For this review, take the finished solid that the model builds, in its own axes (mm). Face numbers are marked on the shaded views. A direction names the side the tool comes from. Coordinates: 2 decimals unless noted, no trailing zeros. Loops run counter-clockwise (first coordinate to the right, second up) from the corner with the lowest first, then second, coordinate; pieces in that order, holes last. Notation, with made-up numbers: (59, 26.5) -> (88, 26.5) arc R28 cw to (88, 64.5) -> close; hole circle Ø9 at (87.25, 18). An arc over 180 degrees is marked (long way). Use a Markdown table: item, result.
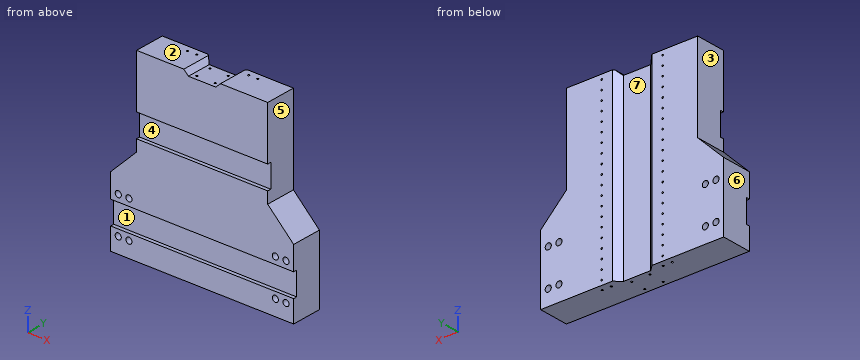
from build123d import *

# Parameters (mm, degrees)
SKETCH1_W                           = 600
SKETCH1_H                           = 600
BOSS_EXTRUDE1_DEPTH                 = 100
CUT_EXTRUDE1_DEPTH                  = 436.889894354
CHAMFER5_SIZE                       = 85
CUT_EXTRUDE2_DEPTH                  = 679.232998313
SKETCH9_R                           = 10
CUT_EXTRUDE5_DEPTH                  = 436.889894354
SKETCH12_R                          = 2.5
CUT_EXTRUDE7_DEPTH                  = 30
SKETCH14_W                          = 90
SKETCH14_H                          = 15
CUT_EXTRUDE8_DEPTH                  = 432.927077179
CHAMFER3_SIZE                       = 15
SKETCH15_W                          = 76.2
SKETCH15_H                          = 12.7
CUT_EXTRUDE9_DEPTH                  = 679.232998313
F_6_0MM_DOWEL_HOLE1_D               = 6
F_6_0MM_DOWEL_HOLE1_DEPTH           = 30
F_6_0MM_DOWEL_HOLE1_TIP             = 1.802581857
F_6_0MM_DOWEL_HOLE1_ON_FACE_2_D     = 6
F_6_0MM_DOWEL_HOLE1_ON_FACE_2_DEPTH = 30
F_6_0MM_DOWEL_HOLE1_ON_FACE_2_TIP   = 1.802581857
F_6_0MM_DOWEL_HOLE1_ON_FACE_3_D     = 6
F_6_0MM_DOWEL_HOLE1_ON_FACE_3_DEPTH = 30
F_6_0MM_DOWEL_HOLE1_ON_FACE_3_TIP   = 1.802581857


with BuildPart() as part:
    # Sketch1 → Boss-Extrude1 (new body)
    with BuildSketch(Plane(origin=(0, 0, 0), x_dir=(1, 0, 0), z_dir=(0, 1, 0))):
        Rectangle(SKETCH1_W, SKETCH1_H)
    extrude(amount=BOSS_EXTRUDE1_DEPTH)

    # Sketch2 → Cut-Extrude1 (cut, through all)
    with BuildSketch(Plane(origin=(0, 100, 0), x_dir=(1, 0, 0), z_dir=(0, 1, 0))):
        Polygon((-300, -300), (-220, -300), (-215, -300), (-215, 74), (-220, 74), (-300, 74), (-300, 60), align=None)
        Polygon((300, -300), (220, -300), (215, -300), (215, 74), (220, 74), (300, 74), (300, 60), align=None)
    extrude(amount=-CUT_EXTRUDE1_DEPTH, mode=Mode.SUBTRACT)

    # Chamfer5
    chamfer5_edges = [part.edges().sort_by_distance(p)[0] for p in [
        (-215, 50, -74),
        (215, 50, -74),
    ]]
    chamfer(chamfer5_edges, length=CHAMFER5_SIZE - 0.0001)  # a hair under: the kernel refuses the full size

    # Sketch3 → Cut-Extrude2 (cut, through all)
    with BuildSketch(Plane.XY.offset(300)):
        Polygon((-35, 81), (-45, 81), (-65, 100), (-45, 100), (45, 100), (65, 100), (45, 81), (35, 81), (0, 81), align=None)
    extrude(amount=-CUT_EXTRUDE2_DEPTH, mode=Mode.SUBTRACT)

    # Sketch9 → Cut-Extrude5 (cut, through all)
    with BuildSketch(Plane(origin=(0, 100, 0), x_dir=(1, 0, 0), z_dir=(0, 1, 0))):
        with Locations(Location((275, 129, 0), (0, 0, 270))):
            Circle(SKETCH9_R)
        with Locations(Location((240, 129, 0), (0, 0, 270))):
            Circle(SKETCH9_R)
        with Locations(Location((240, 249, 0), (0, 0, 270))):
            Circle(SKETCH9_R)
        with Locations(Location((275, 249, 0), (0, 0, 270))):
            Circle(SKETCH9_R)
        with Locations(Location((-275, 129, 0), (0, 0, 90))):
            Circle(SKETCH9_R)
        with Locations(Location((-240, 249, 0), (0, 0, 90))):
            Circle(SKETCH9_R)
        with Locations(Location((-275, 249, 0), (0, 0, 90))):
            Circle(SKETCH9_R)
        with Locations(Location((-240, 129, 0), (0, 0, 90))):
            Circle(SKETCH9_R)
    extrude(amount=-CUT_EXTRUDE5_DEPTH, mode=Mode.SUBTRACT)

    # Sketch12 → Cut-Extrude7 (cut)
    with BuildSketch(Plane(origin=(0, 100, 0), x_dir=(1, 0, 0), z_dir=(0, 1, 0))):
        with Locations(Location((-100, -285, 0), (0, 0, 270))):
            Circle(SKETCH12_R)
        with Locations(Location((100, -285, 0), (0, 0, 270))):
            Circle(SKETCH12_R)
        with Locations(Location((100, -255, 0), (0, 0, 270))):
            Circle(SKETCH12_R)
        with Locations(Location((100, -225, 0), (0, 0, 270))):
            Circle(SKETCH12_R)
        with Locations(Location((100, -195, 0), (0, 0, 270))):
            Circle(SKETCH12_R)
        with Locations(Location((100, -165, 0), (0, 0, 270))):
            Circle(SKETCH12_R)
        with Locations(Location((100, -135, 0), (0, 0, 270))):
            Circle(SKETCH12_R)
        with Locations(Location((100, -105, 0), (0, 0, 270))):
            Circle(SKETCH12_R)
        with Locations(Location((100, -75, 0), (0, 0, 270))):
            Circle(SKETCH12_R)
        with Locations(Location((100, -45, 0), (0, 0, 270))):
            Circle(SKETCH12_R)
        with Locations(Location((100, -15, 0), (0, 0, 270))):
            Circle(SKETCH12_R)
        with Locations(Location((100, 15, 0), (0, 0, 270))):
            Circle(SKETCH12_R)
        with Locations(Location((100, 45, 0), (0, 0, 270))):
            Circle(SKETCH12_R)
        with Locations(Location((100, 75, 0), (0, 0, 270))):
            Circle(SKETCH12_R)
        with Locations(Location((100, 105, 0), (0, 0, 270))):
            Circle(SKETCH12_R)
        with Locations(Location((100, 135, 0), (0, 0, 270))):
            Circle(SKETCH12_R)
        with Locations(Location((100, 165, 0), (0, 0, 270))):
            Circle(SKETCH12_R)
        with Locations(Location((100, 195, 0), (0, 0, 270))):
            Circle(SKETCH12_R)
        with Locations(Location((100, 225, 0), (0, 0, 270))):
            Circle(SKETCH12_R)
        with Locations(Location((100, 255, 0), (0, 0, 270))):
            Circle(SKETCH12_R)
        with Locations(Location((100, 285, 0), (0, 0, 270))):
            Circle(SKETCH12_R)
        with Locations(Location((-100, -255, 0), (0, 0, 270))):
            Circle(SKETCH12_R)
        with Locations(Location((-100, -225, 0), (0, 0, 270))):
            Circle(SKETCH12_R)
        with Locations(Location((-100, -195, 0), (0, 0, 270))):
            Circle(SKETCH12_R)
        with Locations(Location((-100, -165, 0), (0, 0, 270))):
            Circle(SKETCH12_R)
        with Locations(Location((-100, -135, 0), (0, 0, 270))):
            Circle(SKETCH12_R)
        with Locations(Location((-100, -105, 0), (0, 0, 270))):
            Circle(SKETCH12_R)
        with Locations(Location((-100, -75, 0), (0, 0, 270))):
            Circle(SKETCH12_R)
        with Locations(Location((-100, -45, 0), (0, 0, 270))):
            Circle(SKETCH12_R)
        with Locations(Location((-100, -15, 0), (0, 0, 270))):
            Circle(SKETCH12_R)
        with Locations(Location((-100, 15, 0), (0, 0, 270))):
            Circle(SKETCH12_R)
        with Locations(Location((-100, 45, 0), (0, 0, 270))):
            Circle(SKETCH12_R)
        with Locations(Location((-100, 75, 0), (0, 0, 270))):
            Circle(SKETCH12_R)
        with Locations(Location((-100, 105, 0), (0, 0, 270))):
            Circle(SKETCH12_R)
        with Locations(Location((-100, 135, 0), (0, 0, 270))):
            Circle(SKETCH12_R)
        with Locations(Location((-100, 165, 0), (0, 0, 270))):
            Circle(SKETCH12_R)
        with Locations(Location((-100, 195, 0), (0, 0, 270))):
            Circle(SKETCH12_R)
        with Locations(Location((-100, 225, 0), (0, 0, 270))):
            Circle(SKETCH12_R)
        with Locations(Location((-100, 255, 0), (0, 0, 270))):
            Circle(SKETCH12_R)
        with Locations(Location((-100, 285, 0), (0, 0, 270))):
            Circle(SKETCH12_R)
    extrude(amount=-CUT_EXTRUDE7_DEPTH, mode=Mode.SUBTRACT)

    # Sketch14 → Cut-Extrude8 (cut, through all)
    with BuildSketch(Plane(origin=(0, 81, 0), x_dir=(1, 0, 0), z_dir=(0, 1, 0))):
        with Locations((0, -292.5)):
            Rectangle(SKETCH14_W, SKETCH14_H)
    extrude(amount=-CUT_EXTRUDE8_DEPTH, mode=Mode.SUBTRACT)

    # Chamfer3
    chamfer3_edges = [part.edges().sort_by_distance(p)[0] for p in [
        (45, 40.5, 300),
        (-45, 40.5, 300),
    ]]
    chamfer(chamfer3_edges, length=CHAMFER3_SIZE - 0.0001)  # a hair under: the kernel refuses the full size

    # Sketch15 → Cut-Extrude9 (cut, through all)
    with BuildSketch(Plane.ZY.offset(300)):
        with Locations((86.9, 5.65)):
            Rectangle(SKETCH15_W, SKETCH15_H)
        with Locations((-189.9, 5.65)):
            Rectangle(SKETCH15_W, SKETCH15_H)
    extrude(amount=-CUT_EXTRUDE9_DEPTH, mode=Mode.SUBTRACT)

    # Ø6.0mm Dowel Hole1
    with Locations(Plane(origin=(-30, 66, 285), x_dir=(1, 0, 0), z_dir=(0, 0, 1))):
        with Locations((0, 0), (60, 0), (60, -51), (0, -51)):
            Hole(F_6_0MM_DOWEL_HOLE1_D / 2, depth=F_6_0MM_DOWEL_HOLE1_DEPTH)
            with Locations((0, 0, -(F_6_0MM_DOWEL_HOLE1_DEPTH + F_6_0MM_DOWEL_HOLE1_TIP / 2))):  # 118° drill point
                Cone(0, F_6_0MM_DOWEL_HOLE1_D / 2, F_6_0MM_DOWEL_HOLE1_TIP, mode=Mode.SUBTRACT)

    # Ø6.0mm Dowel Hole1 on face 2
    with Locations(Plane(origin=(30, 66, -300), x_dir=(-1, 0, 0), z_dir=(0, 0, -1))):
        with Locations((0, 0), (60, 0), (60, -51), (0, -51), (145, 14), (115, 14), (-55, 14), (-85, 14)):
            Hole(F_6_0MM_DOWEL_HOLE1_ON_FACE_2_D / 2, depth=F_6_0MM_DOWEL_HOLE1_ON_FACE_2_DEPTH)
            with Locations((0, 0, -(F_6_0MM_DOWEL_HOLE1_ON_FACE_2_DEPTH + F_6_0MM_DOWEL_HOLE1_ON_FACE_2_TIP / 2))):  # 118° drill point
                Cone(0, F_6_0MM_DOWEL_HOLE1_ON_FACE_2_D / 2, F_6_0MM_DOWEL_HOLE1_ON_FACE_2_TIP, mode=Mode.SUBTRACT)

    # Ø6.0mm Dowel Hole1 on face 3
    with Locations(Plane(origin=(-85, 80, 300), x_dir=(1, 0, 0), z_dir=(0, 0, 1))):
        with Locations((0, 0), (-30, 0), (170, 0), (200, 0)):
            Hole(F_6_0MM_DOWEL_HOLE1_ON_FACE_3_D / 2, depth=F_6_0MM_DOWEL_HOLE1_ON_FACE_3_DEPTH)
            with Locations((0, 0, -(F_6_0MM_DOWEL_HOLE1_ON_FACE_3_DEPTH + F_6_0MM_DOWEL_HOLE1_ON_FACE_3_TIP / 2))):  # 118° drill point
                Cone(0, F_6_0MM_DOWEL_HOLE1_ON_FACE_3_D / 2, F_6_0MM_DOWEL_HOLE1_ON_FACE_3_TIP, mode=Mode.SUBTRACT)


solid = part.part
(1) Mouldability with a two-part tool opening along X and no side actions: class the marked faces 4, 5, 6 and 7 as pulls with the +X half, pulls with the -X half, needs draft (parallel to the pull), parting line crosses it, or undercut.
Found:
| item | result |
|---|---|
| face 4 | needs draft |
| face 5 | pulls with the +X half |
| face 6 | pulls with the -X half |
| face 7 | undercut |
(2) For line 1 along X through (y, z) = (78, -105); line 2 along Z through (x, y) = (80, 10); line 3 along X through (y, z) = (77, 45), list the stretches that pass through material, from the lowest coordinate up.
Found:
| item | result |
|---|---|
| line 1 | x = -300 to -102.5, -97.5 to 97.5, 102.5 to 300 |
| line 2 | z = -300 to -228, -151.8 to 48.8, 125 to 300 |
| line 3 | x = -215 to -102.5, -97.5 to 97.5, 102.5 to 215 |
(3) Take a section at C-C on x = -185.5. Write out the cut boundary in (y, z).
Found:
| item | result |
|---|---|
| outline | (0, -300) -> (100, -300) -> (100, 300) -> (0, 300) -> (0, 125) -> (12, 125) -> (12, 48.8) -> (0, 48.8) -> (0, -151.8) -> (12, -151.8) -> (12, -228) -> (0, -228) -> close |
(4) Take a section at B-B on x = 19.5. Write out the cut boundary in (y, z).
Found:
| item | result |
|---|---|
| outline | (0, -300) -> (81, -300) -> (81, 285) -> (0, 285) -> (0, 125) -> (12, 125) -> (12, 48.8) -> (0, 48.8) -> (0, -151.8) -> (12, -151.8) -> (12, -228) -> (0, -228) -> close |
(5) For the marked faces 1, 2 and 3, list the 3-axis set-ups (+Z, -Z, +X, -X, +Y, -Y) from which the entire face can be reached by the end or side of a thin tool; tool diameter is ignored.
Found:
| item | result |
|---|---|
| face 1 | +X, -X, -Y |
| face 2 | +Z, +X, -X, +Y, -Y |
| face 3 | +Z, -X, +Y, -Y |
(6) Take a section at A-A on y = 28.5. State how many separate pieces and enclosed holes the cut face has, plus the area to 3 significant figures.
Found:
| item | result |
|---|---|
| separate pieces | 1 |
| enclosed holes | 8 |
| area | 300,000 mm^2 |
(7) Take a section at D-D on x = -258. Write out the cut boundary in (y, z).
Found:
| item | result |
|---|---|
| outline | (0, -300) -> (100, -300) -> (100, -32) -> (0, -32) -> (0, -151.8) -> (12, -151.8) -> (12, -228) -> (0, -228) -> close |
(8) For pin 1 Ø2 at (y, z) = (28, 31) entering from -X; pin 2 Ø2 at (x, y) = (-217, 68) entering from +Z; pin 3 Ø7 at (x, y) = (30, 66) entering from +Z, all flat-tipped, find the tip position at first contact; note any pin that passes through.
Found:
| item | result |
|---|---|
| pin 1 | stops at x = -215 |
| pin 2 | stops at z = 10 |
| pin 3 | stops at z = 285 |
